Model file for the job. Use its own axes, mm. A direction names the side the tool comes from. Round coordinates to 2 decimals unless told otherwise and drop trailing zeros. Loops run counter-clockwise (first coordinate to the right, second up) from the corner with the lowest first, then second, coordinate; pieces in that order, holes last. Notation, with made-up numbers: M 63,-31 L 84,-31 A23 cw 84,-20 Z; hole C 69.5,15.5 d10. An arc over 180 degrees is marked long. Answer in a Markdown table with one row per item.
from build123d import *

# Parameters (mm, degrees)
BASE_R                   = 4.5
BODY_1_DEPTH             = 1.8
THIN_BASE_R              = 4
BODY_THIN_DEPTH          = 2.5
BASE_2_R                 = 4.5
BODY_2_DEPTH             = 0.7
SCREW_HEAD_HOLE_SKETCH_R = 2.775
SCREW_HEAD_HOLE_DEPTH    = 2
F_3_0_3_DIAMETER_HOLE1_D = 3


with BuildPart() as part:
    # base → body 1 (new body)
    with BuildSketch(Plane.XY):
        Circle(BASE_R)
    extrude(amount=BODY_1_DEPTH)

    # thin base → body thin (add)
    with BuildSketch(Plane.XY.offset(1.8)):
        Circle(THIN_BASE_R)
    extrude(amount=BODY_THIN_DEPTH)

    # base 2 → body 2 (add)
    with BuildSketch(Plane.XY.offset(4.3)):
        Circle(BASE_2_R)
    extrude(amount=BODY_2_DEPTH)

    # screw head hole sketch → screw head hole (cut)
    with BuildSketch(Plane.XY.offset(5)):
        Circle(SCREW_HEAD_HOLE_SKETCH_R)
    extrude(amount=-SCREW_HEAD_HOLE_DEPTH, mode=Mode.SUBTRACT)

    # Ø3.0 (3) Diameter Hole1 (through all)
    with Locations(Plane.XY.offset(3)):
        with Locations((0, 0)):
            Hole(F_3_0_3_DIAMETER_HOLE1_D / 2)


solid = part.part
1. Pin check, flat tips, straight feed: pin 1 (1 mm diameter, centred on y = 1.5, z = 2.5, fed in from +X); pin 2 (3 mm diameter, centred on x = -3.5, z = 1.5, fed in from -Y); pin 3 (2.5 mm diameter, centred on x = 0, y = 0, fed in from +Z). Stop position of each tip, or through.
Verdict:
| item | result |
|---|---|
| pin 1 | stops at x = 3.87 |
| pin 2 | stops at y = -4.03 |
| pin 3 | passes through |
2. Saw through at D-D (x = -3). Write the cut outline in (y, z).
Verdict:
| item | result |
|---|---|
| outline | M -3.35,0 L 3.35,0 L 3.35,1.8 L 2.65,1.8 L 2.65,4.3 L 3.35,4.3 L 3.35,5 L -3.35,5 L -3.35,4.3 L -2.65,4.3 L -2.65,1.8 L -3.35,1.8 Z |
3. Mould opens along Y. For faces 1 (the cylindrical face through (-0.867, -3.905, 3.032)), 2 (the cylindrical face through (1.49, 2.34, 4.01)), 3 (the flat face through (0, -3, 5)) say: +Y half, -Y half, draft (parallel to the pull), parting line (faces both ways), or undercut.
Verdict:
| item | result |
|---|---|
| face 1 | parting line |
| face 2 | undercut |
| face 3 | draft |
4. Saw through at A-A (y = 0). Write the cut outline in (x, z) (3 decimals), and give its area (3 significant figures).
Verdict:
| item | result |
|---|---|
| outline | M -4.5,0 L -1.5,0 L -1.5,3 L -2.775,3 L -2.775,5 L -4.5,5 L -4.5,4.3 L -4,4.3 L -4,1.8 L -4.5,1.8 Z; M 1.5,0 L 4.5,0 L 4.5,1.8 L 4,1.8 L 4,4.3 L 4.5,4.3 L 4.5,5 L 2.775,5 L 2.775,3 L 1.5,3 Z |
| area | 22.4 mm² |
5. Tool access for faces 4 (the flat face through (1.2, -1.2, 3)), 5 (the cylindrical face through (1.5, 0.07, 1.48)), 6 (the flat face through (-3, -3, 1.8)): list every direction of +Z, -Z, +X, -X, +Y, -Y with a clear straight run to the whole face (end or side of a thin tool).
Verdict:
| item | result |
|---|---|
| face 4 | +Z |
| face 5 | +Z, -Z |
| face 6 | none |
6. Saw through at C-C (z = 1.65). Write the cut outline in (x, y), and give its area (3 significant figures).
Verdict:
| item | result |
|---|---|
| outline | C 0,0 d9; hole C 0,0 d3 |
| area | 56.5 mm² |
7. Wall check: probe 1 along Y at (x, z) = (0, 0.95); probe 2 along Y at (x, z) = (0, 4.5) (3 decimals); probe 3 along X at (y, z) = (0.5, 3.2). Give the ranges that are in metal, low to high.
Verdict:
| item | result |
|---|---|
| probe 1 | y = -4.5 to -1.5, 1.5 to 4.5 |
| probe 2 | y = -4.5 to -2.775, 2.775 to 4.5 |
| probe 3 | x = -3.97 to -2.73, 2.73 to 3.97 |
